```python
from build123d import *

# Parameters (mm, degrees)
SKETCH_1_W             = 200
SKETCH_1_H             = 200
SM_BASE_FLANGE_1_DEPTH = 10
SKETCH_3_R             = 8
CUT_EXTRUDE_1_DEPTH    = 10


# Sheet-metal steps are written as plain solids
with BuildPart() as part:
    # Sketch 1 → Базовая кромка1 (new body)
    with BuildSketch(Plane.XY):
        with Locations((100, -100)):
            Rectangle(SKETCH_1_W, SKETCH_1_H)
    extrude(amount=-SM_BASE_FLANGE_1_DEPTH)

    # Эскиз3 → Вырез-Вытянуть1 (cut)
    with BuildSketch(Plane(origin=(0, 0, -10), x_dir=(-1, 0, 0), z_dir=(0, 0, -1))):
        with Locations((-175, -100)):
            Circle(SKETCH_3_R)
        with Locations((-100, -25)):
            Circle(SKETCH_3_R)
        with Locations(Location((-25, -100, 0), (0, 0, 180))):
            Circle(SKETCH_3_R)
    extrude(amount=-CUT_EXTRUDE_1_DEPTH, mode=Mode.SUBTRACT)


solid = part.part
```
Input: part model. Units: mm. Frame: model coordinates. Coordinates: 2 decimals unless noted, no trailing zeros. Write each loop counter-clockwise with the first axis right and the second up, starting at its lowest first coordinate (ties: lowest second). Pieces come first, ordered by that corner, then holes. Notation, with made-up numbers: (15, 86) -> (39, 86) arc R11 cw to (39, 93) -> close; hole circle Ø5 at (61.5, 11). An arc over 180 degrees is marked (long way). Write each question's results on one line, items separated by ' | '.
Item 1: Mould query, pull axis X, two halves, no side actions, for faces 1 (the flat face through (99, 0, -5)), 2 (the cylindrical face through (167.61, -103.06, -5.07)), 3 (the flat face through (0, -101, -5)). Classes: +X half, -X half, draft (parallel to the pull), parting line (faces both ways), or undercut.
Conclusion:
face 1: draft | face 2: undercut | face 3: -X half
Item 2: Section query C-C on z = -1.5. Return loops of the section in (x, y), plus the area to 3 significant figures.
Conclusion:
outline: (0, -200) -> (200, -200) -> (200, 0) -> (0, 0) -> close; hole circle Ø16 at (25, -100); hole circle Ø16 at (100, -25); hole circle Ø16 at (175, -100) | area: 39,400 mm^2
Item 3: Section query D-D on y = -100. Return loops of the section in (x, z), plus the area to 3 significant figures.
Conclusion:
outline: (0, -10) -> (17, -10) -> (17, 0) -> (0, 0) -> close; (33, -10) -> (167, -10) -> (167, 0) -> (33, 0) -> close; (183, -10) -> (200, -10) -> (200, 0) -> (183, 0) -> close | area: 1,680 mm^2
Item 4: Section query B-B on y = -25. Return loops of the section in (x, z).
Conclusion:
outline: (0, -10) -> (92, -10) -> (92, 0) -> (0, 0) -> close; (108, -10) -> (200, -10) -> (200, 0) -> (108, 0) -> close
Item 5: Material intervals for probe 1 along Y at (x, z) = (25, -7.75); probe 2 along Y at (x, z) = (174, -7.75); probe 3 along X at (y, z) = (-22, -0.25), sorted ascending.
Conclusion:
probe 1: y = -200 to -108, -92 to 0 | probe 2: y = -200 to -107.94, -92.06 to 0 | probe 3: x = 0 to 92.58, 107.42 to 200
Item 6: Section query A-A on x = 175. Return loops of the section in (y, z), plus the area to 3 significant figures.
Conclusion:
outline: (-200, -10) -> (-108, -10) -> (-108, 0) -> (-200, 0) -> close; (-92, -10) -> (0, -10) -> (0, 0) -> (-92, 0) -> close | area: 1,840 mm^2
Item 7: Pin query (flat end, axial travel): pin 1 Ø13 at (x, y) = (25, -100) entering from -Z. Return the tip coordinate at first contact, or that it passes through.
Conclusion:
pin 1: passes through
